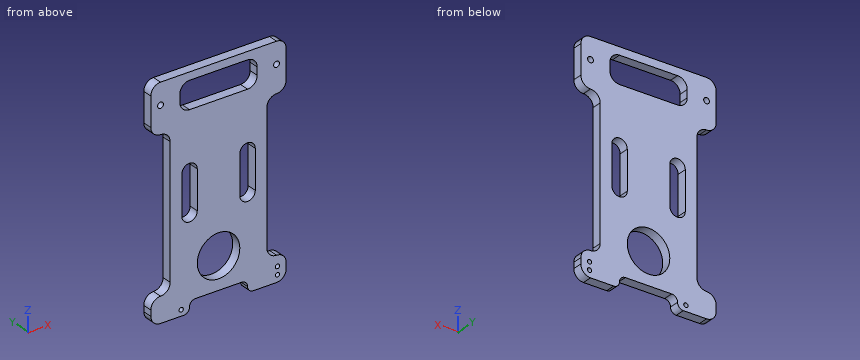
```python
from build123d import *

# Parameters (mm, degrees)
SKETCH_1_W          = 70
SKETCH_1_H          = 115
SKETCH_1_R          = 1.5
SKETCH_1_R_2        = 1.1
SKETCH_1_R_3        = 11
SKETCH_1_W_2        = 40
SKETCH_1_H_2        = 14
EXTRUDE_1_DEPTH     = 5
FILLET_1_R          = 5
FILLET_2_R          = 5
SKETCH_3_W          = 30
SKETCH_3_H          = 6
SKETCH_3_W_2        = 10
SKETCH_3_H_2        = 77
CUT_EXTRUDE_1_DEPTH = 5
FILLET_START        = -1
FILLET_4_DEPTH      = 7
FILLET_4_2_DEPTH    = 5
FILLET_5_R          = 5
CUT_EXTRUDE_2_DEPTH = 10


with BuildPart() as part:
    # 草图1 → 凸台-拉伸1 (new body)
    with BuildSketch(Plane(origin=(0, 0, 0), x_dir=(1, 0, 0), z_dir=(0, 1, 0))):
        Rectangle(SKETCH_1_W, SKETCH_1_H)
        with Locations(Location((30, -46.5, 0), (0, 0, 270))):
            Circle(SKETCH_1_R, mode=Mode.SUBTRACT)
        with Locations(Location((-30, -46.5, 0), (0, 0, 270))):
            Circle(SKETCH_1_R, mode=Mode.SUBTRACT)
        with Locations(Location((30.5, 53.96, 0), (0, 0, 270))):
            Circle(SKETCH_1_R_2, mode=Mode.SUBTRACT)
        with Locations(Location((30.5, 49.96, 0), (0, 0, 270))):
            Circle(SKETCH_1_R_2, mode=Mode.SUBTRACT)
        with Locations(Location((-19.3, 54.46, 0), (0, 0, 270))):
            Circle(SKETCH_1_R_2, mode=Mode.SUBTRACT)
        with Locations(Location((0, 35, 0), (0, 0, 270))):
            Circle(SKETCH_1_R_3, mode=Mode.SUBTRACT)
        with Locations((0, -46.5)):
            Rectangle(SKETCH_1_W_2, SKETCH_1_H_2, mode=Mode.SUBTRACT)
    extrude(amount=EXTRUDE_1_DEPTH)

    # 圆角1
    fillet_1_edges = [part.edges().sort_by_distance(p)[0] for p in [
        (-35, 2.5, 57.5),
        (-35, 2.5, -57.5),
        (35, 2.5, -57.5),
        (35, 2.5, 57.5),
    ]]
    fillet(fillet_1_edges, radius=FILLET_1_R)

    # 圆角2
    fillet_2_edges = [part.edges().sort_by_distance(p)[0] for p in [
        (20, 2.5, 39.5),
        (-20, 2.5, 39.5),
        (-20, 2.5, 53.5),
        (20, 2.5, 53.5),
    ]]
    fillet(fillet_2_edges, radius=FILLET_2_R)

    # 草图3 → 切除-拉伸1 (cut)
    with BuildSketch(Plane(origin=(0, 5, 0), x_dir=(1, 0, 0), z_dir=(0, 1, 0))):
        with Locations((0, 54.5)):
            Rectangle(SKETCH_3_W, SKETCH_3_H)
        with Locations((30, 6)):
            Rectangle(SKETCH_3_W_2, SKETCH_3_H_2)
        with Locations((-30, 6)):
            Rectangle(SKETCH_3_W_2, SKETCH_3_H_2)
    extrude(amount=-CUT_EXTRUDE_1_DEPTH, mode=Mode.SUBTRACT)

    # 圆角4: read off the stored shape, not the designer's step
    # 圆角4 outline → 圆角4 (cut)
    with BuildSketch(Plane(origin=(0, 0, 0), x_dir=(1, 0, 0), z_dir=(0, 1, 0)).offset(FILLET_START)):
        with BuildLine():
            Line((15, 57.5), (15, 54.5))
            ThreePointArc((15, 54.5), (15.878679656, 56.621320344), (18, 57.5))
            Line((18, 57.5), (15, 57.5))
        make_face()
        with BuildLine():
            ThreePointArc((-18, 57.5), (-15.878679656, 56.621320344), (-15, 54.5))
            Line((-15, 54.5), (-15, 57.5))
            Line((-15, 57.5), (-18, 57.5))
        make_face()
    extrude(amount=FILLET_4_DEPTH, mode=Mode.SUBTRACT)

    # Fillet 4 2 outline → Fillet 4 2 (add)
    with BuildSketch(Plane(origin=(0, 0, 0), x_dir=(1, 0, 0), z_dir=(0, 1, 0))):
        with BuildLine():
            Line((15, 51.5), (15, 54.5))
            ThreePointArc((15, 54.5), (14.121320344, 52.378679656), (12, 51.5))
            Line((12, 51.5), (15, 51.5))
        make_face()
        with BuildLine():
            Line((-15, 51.5), (-12, 51.5))
            ThreePointArc((-12, 51.5), (-14.121320344, 52.378679656), (-15, 54.5))
            Line((-15, 54.5), (-15, 51.5))
        make_face()
    extrude(amount=FILLET_4_2_DEPTH)

    # 圆角5
    fillet_5_edges = [part.edges().sort_by_distance(p)[0] for p in [
        (-25, 2.5, 32.5),
        (25, 2.5, 32.5),
        (25, 2.5, -44.5),
        (-25, 2.5, -44.5),
    ]]
    fillet(fillet_5_edges, radius=FILLET_5_R)
    fillet_5_2_edges = [part.edges().sort_by_distance(p)[0] for p in [
        (-35, 2.5, 32.5),
        (35, 2.5, 32.5),
        (35, 2.5, -44.5),
        (-35, 2.5, -44.5),
    ]]
    fillet(fillet_5_2_edges, radius=FILLET_5_R - 0.0001)  # a hair under: the kernel refuses the full size

    # 草图4 → 切除-拉伸2 (cut)
    with BuildSketch(Plane(origin=(0, 5, 0), x_dir=(1, 0, 0), z_dir=(0, 1, 0))):
        with BuildLine():
            Line((11, -10), (11, 10))
            ThreePointArc((11, 10), (15, 14), (19, 10))
            Line((19, 10), (19, -10))
            ThreePointArc((19, -10), (15, -14), (11, -10))
        make_face()
        with BuildLine():
            Line((-11, -10), (-11, 10))
            ThreePointArc((-11, 10), (-15, 14), (-19, 10))
            Line((-19, 10), (-19, -10))
            ThreePointArc((-19, -10), (-15, -14), (-11, -10))
        make_face()
    extrude(amount=-CUT_EXTRUDE_2_DEPTH, mode=Mode.SUBTRACT)


solid = part.part
```
Geometry: final body of the model. Coordinates: model frame, mm. Give positions to 0.01 mm unless a question says otherwise; leave off trailing zeros. Write each loop counter-clockwise with the first axis right and the second up, starting at its lowest first coordinate (ties: lowest second). Pieces come first, ordered by that corner, then holes.
1. Section query A-A, the plane x = 0. Return loops of the section in (y, z), then the cut area to 3 significant figures.
2. Line query: probe 1 along X at (y, z) = (2.7, -3); probe 2 along X at (y, z) = (1.55, 46.5); probe 3 along Z at (x, y) = (2, 4). Output: solid intervals per line, ascending.
3. Section query C-C, the plane y = 2.5. Count the separate pieces of the cut face and the enclosed holes in it, then the cut area to 3 significant figures.
4. Pin query (flat end, axial travel): P1, Ø2.5, axis at y = 2.5, z = 3, coming from the -X side; P2, Ø1.5, axis at y = 2, z = 0, coming from the +X side; P3, Ø2.5, axis at x = -30, z = 46.5, coming from the +Y side. Return the tip coordinate at first contact, or that it passes through.
5. Section query B-B, the plane z = -7. Return loops of the section in (x, y), then the cut area to 3 significant figures.
Computed:
1. outline: (0, -51.5) - (5, -51.5) - (5, -46) - (0, -46) - close; (0, -24) - (5, -24) - (5, 39.5) - (0, 39.5) - close; (0, 53.5) - (5, 53.5) - (5, 57.5) - (0, 57.5) - close
1. area: 365 mm2
2. probe 1: x = -25 to -19, -11 to 11, 19 to 25
2. probe 2: x = -35 to -31.5, -28.5 to -20, 20 to 28.5, 31.5 to 35
2. probe 3: z = -51.5 to -45.82, -24.18 to 39.5, 53.5 to 57.5
3. separate pieces: 1
3. enclosed holes: 9
3. area: 4,940 mm2
4. P1: stops at x = -25
4. P2: stops at x = 25
4. P3: passes through
5. outline: (-25, 0) - (-19, 0) - (-19, 5) - (-25, 5) - close; (-11, 0) - (11, 0) - (11, 5) - (-11, 5) - close; (19, 0) - (25, 0) - (25, 5) - (19, 5) - close
5. area: 170 mm2
